Work out the finished part from the listing and answer in its coordinate system (mm). A direction names the side the tool comes from. Coordinates: 2 decimals unless noted, no trailing zeros. Loops run counter-clockwise (first coordinate to the right, second up) from the corner with the lowest first, then second, coordinate; pieces in that order, holes last. Notation, with made-up numbers: (46, 74) -> (69, 74) arc R28 cw to (69, 95) -> close; hole circle Ø4 at (-24, -17). An arc over 180 degrees is marked (long way). One line per question, with ' | ' between items.
```python
from build123d import *

# Parameters (mm, degrees)
SKETCH1_W               = 112
SKETCH1_H               = 147
BOSS_EXTRUDE1_DEPTH     = 3
SKETCH2_W               = 61
SKETCH2_H               = 61
BOSS_EXTRUDE2_DEPTH     = 3
SKETCH2_2_W             = 61
SKETCH2_2_H             = 61
CUT_EXTRUDE1_DEPTH      = 93.451338552
SKETCH3_R               = 1.75
SKETCH3_R_2             = 2.4
SKETCH3_R_3             = 4.75
SKETCH3_R_4             = 3
SKETCH3_R_5             = 3.5
CUT_EXTRUDE2_DEPTH      = 10
SKETCH4_R               = 2.1
CUT_EXTRUDE3_DEPTH      = 5
MIRROR2_COPY_1_SKETCH_R = 2.1
MIRROR2_COPY_1_DEPTH    = 5
FILLET1_R               = 2
SKETCH5_W               = 37.020085877
SKETCH5_H               = 31.91839976
BOSS_EXTRUDE4_DEPTH     = 1
CHAMFER4_SIZE           = 2.34385688
CHAMFER4_SIZE_2         = 3
MIRROR9_START           = 14.5
MIRROR9_DEPTH           = 16
MIRROR9_START_2         = 7
MIRROR9_2_DEPTH         = 1.838834765
FILLET2_R               = 5


with BuildPart() as part:
    # Sketch1 → Boss-Extrude1 (new body)
    with BuildSketch(Plane(origin=(0, 0, 0), x_dir=(1, 0, 0), z_dir=(0, 1, 0))):
        Rectangle(SKETCH1_W, SKETCH1_H)
    extrude(amount=BOSS_EXTRUDE1_DEPTH)

    # Sketch2 → Boss-Extrude2 (add)
    with BuildSketch(Plane(origin=(0, 3, 0), x_dir=(1, 0, 0), z_dir=(0, 1, 0))):
        with Locations((0, 37)):
            Rectangle(SKETCH2_W, SKETCH2_H)
    extrude(amount=-BOSS_EXTRUDE2_DEPTH)

    # Sketch2<2> → Cut-Extrude1 (cut, through all)
    with BuildSketch(Plane(origin=(0, 3, 0), x_dir=(1, 0, 0), z_dir=(0, 1, 0))):
        with Locations((0, 37)):
            Rectangle(SKETCH2_2_W, SKETCH2_2_H)
    extrude(amount=-CUT_EXTRUDE1_DEPTH, mode=Mode.SUBTRACT)

    # Sketch3 → Cut-Extrude2 (cut)
    with BuildSketch(Plane(origin=(0, 3, 0), x_dir=(1, 0, 0), z_dir=(0, 1, 0))):
        with Locations(Location((12.415, -18.57, 0), (0, 0, 270))):
            Circle(SKETCH3_R)
        with Locations(Location((28.345, -18.57, 0), (0, 0, 270))):
            Circle(SKETCH3_R)
        with Locations(Location((-41.010240817, -44.763305049, 0), (0, 0, 270))):
            Circle(SKETCH3_R_2)
        with Locations(Location((-41.010240817, -56.907347776, 0), (0, 0, 270))):
            Circle(SKETCH3_R_2)
        with Locations(Location((-23.966529419, -15.947077361, 0), (0, 0, 270))):
            Circle(SKETCH3_R_2)
        with Locations(Location((-7, -36.196378326, 0), (0, 0, 270))):
            Circle(SKETCH3_R_3)
        with Locations(Location((19.612753758, -52.279000863, 0), (0, 0, 270))):
            Circle(SKETCH3_R_4)
        with Locations(Location((37.612753758, -52.279000863, 0), (0, 0, 270))):
            Circle(SKETCH3_R_4)
        with Locations(Location((-41.753496243, -15.947077361, 0), (0, 0, 270))):
            Circle(SKETCH3_R_5)
    extrude(amount=-CUT_EXTRUDE2_DEPTH, mode=Mode.SUBTRACT)

    # Sketch4 → Cut-Extrude3 (cut)
    with BuildSketch(Plane(origin=(0, 3, 0), x_dir=(1, 0, 0), z_dir=(0, 1, 0))):
        with Locations(Location((-52, -69.5, 0), (0, 0, 270))):
            Circle(SKETCH4_R)
    cut_extrude3 = extrude(amount=-CUT_EXTRUDE3_DEPTH, mode=Mode.SUBTRACT)

    # Mirror1: Cut-Extrude3 across plane
    add(cut_extrude3.mirror(Plane(origin=(0, 0, 0), x_dir=(0, 0, 1), z_dir=(1, 0, 0))), mode=Mode.SUBTRACT)

    # Mirror2: Cut-Extrude3 across plane
    add(cut_extrude3.mirror(Plane.XY), mode=Mode.SUBTRACT)

    # Mirror2 copy 1 sketch → Mirror2 copy 1 (cut)
    with BuildSketch(Plane(origin=(0, 3, 0), x_dir=(-1, 0, 0), z_dir=(0, 1, 0))):
        with Locations(Location((-52, -69.5, 0), (0, 0, 270))):
            Circle(MIRROR2_COPY_1_SKETCH_R)
    extrude(amount=-MIRROR2_COPY_1_DEPTH, mode=Mode.SUBTRACT)

    # Fillet1
    fillet1_edges = [part.edges().sort_by_distance(p)[0] for p in [
        (56, 1.5, 73.5),
        (-56, 1.5, 73.5),
        (-56, 1.5, -73.5),
        (56, 1.5, -73.5),
    ]]
    fillet(fillet1_edges, radius=FILLET1_R)

    # Sketch5 → Boss-Extrude4 (add)
    with BuildSketch(Plane(origin=(0, 2, 0), x_dir=(1, 0, 0), z_dir=(0, 1, 0))):
        with Locations((-29.010042938, 15.54080012)):
            Rectangle(SKETCH5_W, SKETCH5_H)
    extrude(amount=BOSS_EXTRUDE4_DEPTH)

    # Chamfer1
    # the kernel refuses this chamfer: 5 mm, written as the material it takes off along each edge
    with BuildSketch(Plane(origin=(-10.5, 3, -44.35841494), x_dir=(-1, 0, 0), z_dir=(0, 0, 1))) as chamfer1_piece_1:
        with BuildLine():
            Line((5.141421356, -0.141421356), (-0.141421356, 5.141421356))
            Line((-0.141421356, 5.141421356), (-0.241421356, 5.141421356))
            ThreePointArc((-0.241421356, 5.141421356), (-0.1, 2.570710678), (-0.1, 0))
            Line((-0.1, 0), (0, -0.1))
            ThreePointArc((0, -0.1), (2.570710678, -0.1), (5.141421356, -0.241421356))
            Line((5.141421356, -0.241421356), (5.141421356, -0.141421356))
        make_face()
    extrude(amount=37.85841494, mode=Mode.SUBTRACT)

    # Chamfer4
    # the kernel refuses this chamfer: 3, 2.34385688 mm, written as the material it takes off along each edge
    with BuildSketch(Plane(origin=(-30.5, 3, -31.5), x_dir=(0, 0, 1), z_dir=(1, 0, 0))) as chamfer4_piece_1:
        Polygon((CHAMFER4_SIZE, 0), (0, CHAMFER4_SIZE_2), (0, 0), align=None)
    extrude(amount=22.738607652, mode=Mode.SUBTRACT)

    # Mirror9: read off the stored shape, not the designer's step
    # Mirror9 outline → Mirror9 (add)
    with BuildSketch(Plane.YZ.offset(MIRROR9_START)):
        Polygon((2, -29.937428747), (3, -29.15614312), (3, -6.5), (2, -6.5), align=None)
    extrude(amount=MIRROR9_DEPTH)

    # Mirror9 2 outline → Mirror9 2 (cut)
    with BuildSketch(Plane(origin=(0, 0, 0), x_dir=(0.7071067811865509, 0.707106781186544, 0), z_dir=(0.707106781186544, -0.707106781186551, 0)).offset(MIRROR9_START_2)):
        Polygon((13.081475452, -29.15614312), (13.081475452, -6.5), (11.66726189, -6.5), (11.66726189, -29.937428747), align=None)
    extrude(amount=MIRROR9_2_DEPTH, mode=Mode.SUBTRACT)

    # Fillet2
    # the kernel refuses this fillet: 5 mm, written as the material it adds along each edge
    with BuildSketch(Plane(origin=(-30.5, 12.850134419, -21.460374677), x_dir=(1, 0, 0), z_dir=(0, -0.788010753545573, -0.6156614754039254))) as fillet2_piece_1_section:
        with BuildLine():
            CenterArc((FILLET2_R, -FILLET2_R), FILLET2_R, 90, 90)
            Line((0, -FILLET2_R), (0, 0))
            Line((0, 0), (FILLET2_R, 0))
        make_face()
    fillet2_piece_1 = extrude(amount=26.269018215, mode=Mode.PRIVATE)
    fillet2_piece_1 = split(fillet2_piece_1, bisect_by=Plane(origin=(-30.5, 3, -21.460374677), z_dir=(0, -1, 0)), keep=Keep.TOP, mode=Mode.PRIVATE)
    fillet2_piece_1 = split(fillet2_piece_1, bisect_by=Plane(origin=(-30.5, 2, -21.460374677), z_dir=(0, 1, 0)), keep=Keep.TOP, mode=Mode.PRIVATE)
    add(fillet2_piece_1)
    with BuildSketch(Plane(origin=(30.5, -7.850134418, -37.633197192), x_dir=(0, 0.6156614755670328, -0.7880107534181395), z_dir=(0, 0.7880107534181395, 0.6156614755670328))) as fillet2_piece_2_section:
        with BuildLine():
            CenterArc((FILLET2_R, FILLET2_R), FILLET2_R, 180, 90)
            Line((0, FILLET2_R), (0, 0))
            Line((0, 0), (FILLET2_R, 0))
        make_face()
    fillet2_piece_2 = extrude(amount=26.269018215, mode=Mode.PRIVATE)
    fillet2_piece_2 = split(fillet2_piece_2, bisect_by=Plane(origin=(30.5, 3, -37.633197192), z_dir=(0, -1, 0)), keep=Keep.TOP, mode=Mode.PRIVATE)
    fillet2_piece_2 = split(fillet2_piece_2, bisect_by=Plane(origin=(30.5, 2, -37.633197192), z_dir=(0, 1, 0)), keep=Keep.TOP, mode=Mode.PRIVATE)
    add(fillet2_piece_2)


solid = part.part
```
1) For faces 1 (the face through (23, 2, -18)), 2 (the face through (0, 2, -67.5)), 3 (the face through (29.023, 2.298, -31.547)), determine the directions among +Z, -Z, +X, -X, +Y, -Y from which every point of the face is accessible in a straight line to the end or side of a thin tool.
Check values:
face 1: -Y | face 2: +Y, -Y | face 3: +Y
2) Find section B-B (z = 69.5). Write down the section's boundary in (x, y).
Check values:
outline: (-56, 0) -> (-54.1, 0) -> (-54.1, 3) -> (-56, 3) -> close; (-49.9, 0) -> (49.9, 0) -> (49.9, 3) -> (-49.9, 3) -> close; (54.1, 0) -> (56, 0) -> (56, 3) -> (54.1, 3) -> close
3) Find the intervals of material crossed by line 1 along Z through (x, y) = (52, 1.4); line 2 along X through (y, z) = (1.35, -69.5); line 3 along X through (y, z) = (0.65, -8.5), in increasing order.
Check values:
line 1: z = -73.5 to -71.6, -67.4 to 67.4, 71.6 to 73.5 | line 2: x = -56 to -54.1, -49.9 to 49.9, 54.1 to 56 | line 3: x = -56 to -30.5, 30.5 to 56
4) Find section C-C (z = -47). Write down the section's boundary in (x, y).
Check values:
outline: (-56, 0) -> (-30.5, 0) -> (-30.5, 3) -> (-56, 3) -> close; (30.5, 0) -> (56, 0) -> (56, 3) -> (30.5, 3) -> close
5) Find section A-A (x = -52). Write down the section's boundary in (y, z).
Check values:
outline: (0, -73.5) -> (3, -73.5) -> (3, -71.6) -> (0, -71.6) -> close; (0, -67.4) -> (3, -67.4) -> (3, 67.4) -> (0, 67.4) -> close; (0, 71.6) -> (3, 71.6) -> (3, 73.5) -> (0, 73.5) -> close
6) Flat-ended cylindrical pins translate along their axes: pin 1 (4.5 mm diameter, centred on x = -41.01, z = 44.76, fed in from -Y); pin 2 (12 mm diameter, centred on x = 9, z = -14, fed in from +Y). Find the tip coordinate at first contact, or state that the pin passes through.
Check values:
pin 1: passes through | pin 2: stops at y = 2.5
7) Find section D-D (y = 1.5). State how many separate pieces and enclosed holes the cut face has, plus the area to 3 significant figures.
Check values:
separate pieces: 1 | enclosed holes: 14 | area: 12,400 mm^2
8) The mould has two halves that part along X. Classify faces 4 (the face through (-1, 1, -73.5)), 5 (the face through (-29.023, 2.317, -31.532)), 6 (the face through (-56, 1, 1)): released by +X, released by -X, zero draft, split by the parting line, or undercut.
Check values:
face 4: zero draft | face 5: undercut | face 6: released by -X
